Verification items for the finished model (mm, model axes). A direction names the side the tool comes from. Round coordinates to 2 decimals unless told otherwise and drop trailing zeros. Loops run counter-clockwise (first coordinate to the right, second up) from the corner with the lowest first, then second, coordinate; pieces in that order, holes last. Notation, with made-up numbers: (7.25, 42.5) -> (41.25, 42.5) arc R28 ccw to (41.25, 81.5) -> close; hole circle Ø7 at (50.5, 9.25). An arc over 180 degrees is marked (long way). Write item = value, one per line.
Autodesk Inventor part; units mm, degrees
ref_plane "YZ Plane" through (0, 0, 0) normal (1, 0, 0) x (0, 1, 0)
ref_plane "XZ Plane" through (0, 0, 0) normal (0, 1, 0) x (-1, 0, 0)
ref_plane "XY Plane" through (0, 0, 0) normal (0, 0, 1) x (1, 0, 0)
sketch "Sketch1" plane through (0, 0, 0) normal (0, 1, 0) x (-1, 0, 0)
  line L0 (21.2, 0) -> (21.2, -3)
  line L1 (42.4, 0) -> (42.4, -3)
  line L2 (63.6, 0) -> (63.6, -3)
  line L3 (84.8, 0) -> (84.8, -3)
  line L4 (84.8, 0) -> (106, 0)
  line L5 (0, 0) -> (21.2, 0)
  line L6 (42.4, 0) -> (63.6, 0)
  line L7 (21.2, -3) -> (42.4, -3)
  line L8 (63.6, -3) -> (84.8, -3)
  line L9 (106, -21.2) -> (103, -21.2)
  line L10 (106, -42.4) -> (103, -42.4)
  line L11 (106, -63.6) -> (103, -63.6)
  line L12 (106, -84.8) -> (103, -84.8)
  line L13 (106, -84.8) -> (106, -106)
  line L14 (103, -21.2) -> (103, -42.4)
  line L15 (103, -63.6) -> (103, -84.8)
  line L16 (106, 0) -> (106, -21.2)
  line L17 (106, -42.4) -> (106, -63.6)
  line L18 (0, -21.2) -> (3, -21.2)
  line L19 (0, -42.4) -> (3, -42.4)
  line L20 (0, -63.6) -> (3, -63.6)
  line L21 (0, -84.8) -> (3, -84.8)
  line L22 (0, -21.2) -> (0, 0)
  line L23 (3, -84.8) -> (3, -63.6)
  line L24 (3, -42.4) -> (3, -21.2)
  line L25 (0, -106) -> (0, -84.8)
  line L26 (0, -63.6) -> (0, -42.4)
  line L27 (21.2, -106) -> (21.2, -103)
  line L28 (42.4, -106) -> (42.4, -103)
  line L29 (63.6, -106) -> (63.6, -103)
  line L30 (84.8, -106) -> (84.8, -103)
  line L31 (21.2, -106) -> (0, -106)
  line L32 (84.8, -103) -> (63.6, -103)
  line L33 (42.4, -103) -> (21.2, -103)
  line L34 (106, -106) -> (84.8, -106)
  line L35 (63.6, -106) -> (42.4, -106)
  dimension "d0" = 106
  dimension "d1" = 106
extrude "Extrusion1" add sketch "Sketch1" along normal blind 3
sketch "Sketch2" plane through (0, 3, 0) normal (0, 1, 0) x (1, 0, 0)
  circle A0 centre (-25, 20) radius 0.5
  circle A1 centre (-53, 20) radius 0.5
  circle A2 centre (-81, 20) radius 0.5
  circle A3 centre (-81, 53) radius 0.5
  circle A4 centre (-81, 86) radius 0.5
  circle A5 centre (-53, 53) radius 0.5
  circle A6 centre (-53, 86) radius 0.5
  circle A7 centre (-25, 53) radius 0.5
  circle A8 centre (-25, 86) radius 0.5
  point P0 (0, 0)
  dimension "d6" = 1
  dimension "d7" = 1
  dimension "d8" = 1
  dimension "d9" = 1
  dimension "d10" = 1
  dimension "d11" = 1
  dimension "d12" = 1
  dimension "d13" = 1
  dimension "d14" = 1
hole "Hole1" at (-81, 3, -20) direction (0, -1, 0) diameter 3 end through all
sketch "Sketch3" plane through (0, 3, 0) normal (0, 1, 0) x (1, 0, 0)
  line L0 (-21.2, 0) -> (0, 0)
  line L1 (0, 0) -> (-106, 0)
  line L2 (-106, 0) -> (-106, 106)
  line L3 (-106, 106) -> (0, 106)
  line L4 (0, 106) -> (0, 0)
  line L5 (3, -3) -> (-109, -3)
  line L6 (-109, -3) -> (-109, 109)
  line L7 (-109, 109) -> (3, 109)
  line L8 (3, 109) -> (3, -3)
  dimension "d22" = 112
  dimension "d23" = 112
extrude "Extrusion2" add sketch "Sketch3" against normal blind 3
sketch "Sketch5" plane through (0, 0, 0) normal (0, -1, 0) x (1, 0, 0)
  circle A0 centre (-25, -20) radius 1.5
  point P0 (0, 0)
  dimension "d26" = 3
hole "Hole2" at (-25, 0, -20) direction (0, 1, 0) diameter 3 end through all
sketch "Sketch6" plane through (0, 0, 0) normal (0, -1, 0) x (1, 0, 0)
  circle A0 centre (-25, -53) radius 1.5
  point P0 (0, 0)
  dimension "d34" = 3
hole "Hole3" at (-25, 0, -53) direction (0, 1, 0) diameter 3 end through all
sketch "Sketch7" plane through (0, 0, 0) normal (0, -1, 0) x (1, 0, 0)
  circle A0 centre (-53, -20) radius 1.5
  point P0 (0, 0)
  dimension "d42" = 3
hole "Hole4" at (-53, 0, -20) direction (0, 1, 0) diameter 3 end through all
sketch "Sketch8" plane through (0, 0, 0) normal (0, -1, 0) x (1, 0, 0)
  circle A0 centre (-53, -53) radius 1.5
  point P0 (0, 0)
  dimension "d50" = 3
hole "Hole5" at (-53, 0, -53) direction (0, 1, 0) diameter 3 end through all
sketch "Sketch9" plane through (0, 0, 0) normal (0, -1, 0) x (1, 0, 0)
  circle A0 centre (-25, -86) radius 1.5
  point P0 (0, 0)
  dimension "d58" = 3
hole "Hole6" at (-25, 0, -86) direction (0, 1, 0) diameter 3 end through all
sketch "Sketch10" plane through (0, 0, 0) normal (0, -1, 0) x (1, 0, 0)
  circle A0 centre (-53, -86) radius 1.5
  point P0 (0, 0)
  dimension "d66" = 3
hole "Hole7" at (-53, 0, -86) direction (0, 1, 0) diameter 3 end through all
sketch "Sketch11" plane through (0, 0, 0) normal (0, -1, 0) x (1, 0, 0)
  circle A0 centre (-81, -53) radius 1.5
  point P0 (0, 0)
  dimension "d74" = 3
hole "Hole8" at (-81, 0, -53) direction (0, 1, 0) diameter 3 end through all
sketch "Sketch12" plane through (0, 0, 0) normal (0, -1, 0) x (1, 0, 0)
  circle A0 centre (-81, -86) radius 1.5
  point P0 (0, 0)
  dimension "d82" = 3
hole "Hole9" at (-81, 0, -86) direction (0, 1, 0) diameter 3 end through all
properties part number "Box top" material "PMMA Plastic"
(1) Sectioned sample at C-C, the plane z = -25.5. Record the cut outline in (x, y).
Filled sheet:
outline = (-109, 0) -> (-106, 0) -> (-106, 3) -> (-109, 3) -> close; (-103, 0) -> (-3, 0) -> (-3, 3) -> (-103, 3) -> close; (0, 0) -> (3, 0) -> (3, 3) -> (0, 3) -> close
(2) Material ranges on probe 1 along X at (y, z) = (1.35, -53); probe 2 along Z at (x, y) = (-25, 1); probe 3 along X at (y, z) = (0.5, -64.5), recorded low to high. Write a range as from..to.
Filled sheet:
probe_1 = -109..-82.5, -79.5..-54.5, -51.5..-26.5, -23.5..3
probe_2 = -109..-106, -103..-87.5, -84.5..-54.5, -51.5..-21.5, -18.5..-3, 0..3
probe_3 = -109..-106, -103..-3, 0..3
(3) Sectioned sample at D-D, the plane x = -25. Record the cut outline in (y, z).
Filled sheet:
outline = (0, -109) -> (3, -109) -> (3, -106) -> (0, -106) -> close; (0, -103) -> (3, -103) -> (3, -87.5) -> (0, -87.5) -> close; (0, -84.5) -> (3, -84.5) -> (3, -54.5) -> (0, -54.5) -> close; (0, -51.5) -> (3, -51.5) -> (3, -21.5) -> (0, -21.5) -> close; (0, -18.5) -> (3, -18.5) -> (3, -3) -> (0, -3) -> close; (0, 0) -> (3, 0) -> (3, 3) -> (0, 3) -> close
(4) Go/stop test with a flat-tipped pin: pin 1 Ø8 at (x, z) = (-23, -66) entering from -Y. Record where the tip stops, or that it passes through.
Filled sheet:
pin_1 = 0
(5) Sectioned sample at B-B, the plane z = -53. Record the cut outline in (x, y).
Filled sheet:
outline = (-109, 0) -> (-82.5, 0) -> (-82.5, 3) -> (-109, 3) -> close; (-79.5, 0) -> (-54.5, 0) -> (-54.5, 3) -> (-79.5, 3) -> close; (-51.5, 0) -> (-26.5, 0) -> (-26.5, 3) -> (-51.5, 3) -> close; (-23.5, 0) -> (3, 0) -> (3, 3) -> (-23.5, 3) -> close
(6) Set-up check for faces 4 (the face through (-1, 1, -42.4)), 5 (the face through (3, 2, -54)): record each of +Z, -Z, +X, -X, +Y, -Y from which the full face is reachable in a straight line by a thin tool's end or side.
Filled sheet:
face_4 = +Y, -Y
face_5 = +Z, -Z, +X, +Y, -Y
(7) Draft check along X on faces 1 (the face through (-54, 0, -41)), 2 (the face through (-74, 1, -3)), 3 (the face through (-109, 2, -52)). Enter one of: released by +X, released by -X, zero draft, split by the parting line, or undercut.
Filled sheet:
face_1 = zero draft
face_2 = undercut
face_3 = released by -X
(8) Sectioned sample at A-A, the plane x = -53. Record the cut outline in (y, z).
Filled sheet:
outline = (0, -109) -> (3, -109) -> (3, -87.5) -> (0, -87.5) -> close; (0, -84.5) -> (3, -84.5) -> (3, -54.5) -> (0, -54.5) -> close; (0, -51.5) -> (3, -51.5) -> (3, -21.5) -> (0, -21.5) -> close; (0, -18.5) -> (3, -18.5) -> (3, 3) -> (0, 3) -> close
